Autodesk Inventor part; units mm, degrees
ref_plane "XZ Plane" through (0, 0, 0) normal (0, 1, 0) x (-1, 0, 0)
sketch "Sketch1" plane through (0, 0, 0) normal (0, 1, 0) x (-1, 0, 0)
  circle A0 centre (0, 0) radius 12.5
  dimension "d0" = 25
extrude "Extrusion1" add sketch "Sketch1" along normal blind 0.9
sketch "Sketch2" plane through (0, 0, 0) normal (0, -1, 0) x (1, 0, 0)
  circle A0 centre (0, 0) radius 39.6
  dimension "d3" = 79.2
extrude "Extrusion2" add sketch "Sketch2" along normal blind 52.5
sketch "Sketch3" plane through (0, 0.9, 0) normal (0, 1, 0) x (1, 0, 0)
  line L0 (0, 0) -> (-9, 0) construction
  circle A0 centre (0, 0) radius 9 construction
  point P0 (-2.7812, -8.5595)
  point P1 (7.2812, -5.2901)
  point P2 (7.2812, 5.2901)
  point P3 (-2.7812, 8.5595)
  point P4 (-2.7812, 8.5595)
  point P5 (7.2812, 5.2901)
  point P6 (7.2812, -5.2901)
  point P7 (-2.7812, -8.5595)
  dimension "d6" = 18
  dimension "d9" = 360
hole "Hole2" at (-9, 0.9, 0) at (-2.7812, 0.9, -8.5595) at (7.2812, 0.9, -5.2901) at (7.2812, 0.9, 5.2901) at (-2.7812, 0.9, 8.5595) direction (0, -1, 0) diameter 3.242 end through all countersink diameter 4 countersink angle 90
sketch "Sketch4" plane through (0, 0, 0) normal (0, 0, 1) x (1, 0, 0)
  line L0 (18.2808, -210.8501) -> (-19.3069, -224.5309)
  line L1 (-19.3069, -224.5309) -> (-18.2808, -227.3499)
  line L2 (-18.2808, -227.3499) -> (19.3069, -213.6691)
  line L3 (19.3069, -213.6691) -> (18.2808, -210.8501)
  line L4 (18.2808, -210.8501) -> (-18.2808, -227.3499) construction
  line L5 (-19.3069, -224.5309) -> (19.3069, -213.6691) construction
  line L6 (12.5, 0.9) -> (-12.5, 0.9) construction
  line L7 (0, 0.9) -> (0, -219.1) construction
  point P0 (0, 0)
  dimension "d25" = 40
  dimension "d27" = 3
  dimension "d28" = 70
  dimension "d29" = 220
sketch "Sketch5" plane through (19.3069, -213.6691, -20) normal (0.342, -0.9397, 0) x (0.9397, 0.342, 0)
  line L0 (0, 0) -> (0, 40)
  line L1 (0, 20) -> (-20, 20) construction
  line L2 (-20, 20) -> (-20, 0) construction
  line L3 (0, 0) -> (-40, 0)
  circle A0 centre (-20, 20) radius 15
  point P0 (54.9366, 20)
  dimension "d32" = 30
properties part number "CH_01_0044_motor_end"
Read the model definition and answer for the solid it produces. Units are mm, in the model's axes. A direction names the side the tool comes from. Coordinates: 2 decimals unless noted, no trailing zeros. Loops run counter-clockwise (first coordinate to the right, second up) from the corner with the lowest first, then second, coordinate; pieces in that order, holes last. Notation, with made-up numbers: (47.25, 68.5) - (72.25, 68.5) arc R22 cw to (72.25, 83.5) - close; hole circle Ø10 at (27.5, -21.5). An arc over 180 degrees is marked (long way). Answer in a Markdown table with one row per item.
Q1. Find section D-D on z = -29.5. Write down the section's boundary in (x, y).
Here are the results:
| item | result |
|---|---|
| outline | (-26.42, -52.5) - (26.42, -52.5) - (26.42, 0) - (-26.42, 0) - close |
Q2. Find section A-A on z = 0. Write down the section's boundary in (x, y), plus the area to 3 significant figures.
Here are the results:
| item | result |
|---|---|
| outline | (-39.6, -52.5) - (-10.62, -52.5) - (-10.62, 0.52) - (-11, 0.9) - (-12.5, 0.9) - (-12.5, 0) - (-39.6, 0) - close; (-7.38, -52.5) - (39.6, -52.5) - (39.6, 0) - (12.5, 0) - (12.5, 0.9) - (-7, 0.9) - (-7.38, 0.52) - close |
| area | 4,010 mm^2 |
Q3. The mould has two halves that part along Z. Classify faces 3 (the cylindrical face through (-4.15, -26.36, -7.69)), 4 (the cylindrical face through (-11.923, 0.444, -3.755)), 5 (the flat face through (-1, -52.5, 1)), 6 (the cylindrical face through (-10.607, -26.361, -0.211)): pulls with the +Z half, pulls with the -Z half, needs draft (parallel to the pull), parting line crosses it, or undercut.
Here are the results:
| item | result |
|---|---|
| face 3 | undercut |
| face 4 | parting line crosses it |
| face 5 | needs draft |
| face 6 | undercut |
Q4. Given P1, Ø10, axis at x = -4.5, y = -21.5, coming from the -Z side; P2, Ø8, axis at x = 23, y = -12.5, coming from the -Z side; P3, Ø4, axis at y = -35.5, z = 14, coming from the -X side, each flat-ended and moving along its own axis, determine where each tip first touches the part or whether it passes through.
Here are the results:
| item | result |
|---|---|
| P1 | stops at z = -39.6 |
| P2 | stops at z = -34.74 |
| P3 | stops at x = -37.74 |
Q5. Find section C-C on y = -25.5. Write down the section's boundary in (x, z).
Here are the results:
| item | result |
|---|---|
| outline | circle Ø79.2 at (0, 0); hole circle Ø3.24 at (-9, 0); hole circle Ø3.24 at (-2.78, -8.56); hole circle Ø3.24 at (-2.78, 8.56); hole circle Ø3.24 at (7.28, -5.29); hole circle Ø3.24 at (7.28, 5.29) |
Q6. Find section B-B on x = -9. Write down the section's boundary in (y, z).
Here are the results:
| item | result |
|---|---|
| outline | (-52.5, -38.56) - (0, -38.56) - (0, -8.67) - (0.9, -8.67) - (0.9, -2) - (0.52, -1.62) - (-52.5, -1.62) - close; (-52.5, 1.62) - (0.52, 1.62) - (0.9, 2) - (0.9, 8.67) - (0, 8.67) - (0, 38.56) - (-52.5, 38.56) - close |
Q7. For faces 1 (the cylindrical face through (-2.16, -26.361, 10.057)), 2 (the flat face through (-9, 0, 9)), determine the directions among +Z, -Z, +X, -X, +Y, -Y from which every point of the face is accessible in a straight line to the end or side of a thin tool.
Here are the results:
| item | result |
|---|---|
| face 1 | +Y, -Y |
| face 2 | +Y |
Q8. Straight lines are drawn through the part: line 1 along Y through (x, z) = (35, 14); line 2 along Z through (x, y) = (-9, -19); line 3 along Z through (x, y) = (30.5, -14). For each, find the intervals that lie inside material, in ascending order. Write a range as [from, to].
Here are the results:
| item | result |
|---|---|
| line 1 | y = [-52.5, 0] |
| line 2 | z = [-38.56, -1.62], [1.62, 38.56] |
| line 3 | z = [-25.26, 25.26] |
